Geometry: final body of the model. Coordinates: model frame, mm. A direction names the side the tool comes from. Give positions to 0.01 mm unless a question says otherwise; leave off trailing zeros. Write each loop counter-clockwise with the first axis right and the second up, starting at its lowest first coordinate (ties: lowest second). Pieces come first, ordered by that corner, then holes.
```python
from build123d import *

# Parameters (mm, degrees)
BOSS_EXTRU_1_DEPTH      = 6
ESQUISSE2_W             = 150
ESQUISSE2_H             = 120
BOSS_EXTRU_2_DEPTH      = 6
ESQUISSE3_W             = 6
ESQUISSE3_H             = 50
ESQUISSE3_W_2           = 50
ESQUISSE3_H_2           = 6
ENL_V_MAT_EXTRU_1_DEPTH = 10
ESQUISSE4_W             = 50
ESQUISSE4_H             = 6
ENL_V_MAT_EXTRU_2_DEPTH = 10
ESQUISSE5_W             = 263.306064462
ESQUISSE5_H             = 531.54399855
ENL_V_MAT_EXTRU_5_DEPTH = 10
ESQUISSE9_W             = 6
ESQUISSE9_H             = 75
ESQUISSE9_H_2           = 50
ESQUISSE9_H_3           = 40
ENL_V_MAT_EXTRU_6_DEPTH = 10


with BuildPart() as part:
    # Esquisse1 → Boss.-Extru.1 (new body)
    with BuildSketch(Plane.XY):
        Polygon((-50, 335.901139534), (50, 335.901139534), (255.775862069, 10.507079064), (205, -75.642859016), (-205, -75.642859016), (-255.775862069, 10.507079064), align=None)
        with BuildLine():
            Line((-189.319805153, 31.819805153), (-191.794678888, 34.294678888))
            ThreePointArc((-191.794678888, 34.294678888), (-206, 0), (-191.794678888, -34.294678888))
            Line((-191.794678888, -34.294678888), (-189.319805153, -31.819805153))
            ThreePointArc((-189.319805153, -31.819805153), (-202.5, 0), (-189.319805153, 31.819805153))
        make_face(mode=Mode.SUBTRACT)
        with BuildLine():
            Line((-125.680194847, 31.819805153), (-123.205321112, 34.294678888))
            ThreePointArc((-123.205321112, 34.294678888), (-109, 0), (-123.205321112, -34.294678888))
            Line((-123.205321112, -34.294678888), (-125.680194847, -31.819805153))
            ThreePointArc((-125.680194847, -31.819805153), (-112.5, 0), (-125.680194847, 31.819805153))
        make_face(mode=Mode.SUBTRACT)
        with BuildLine():
            Line((-84.319805153, -31.819805153), (-86.794678888, -34.294678888))
            ThreePointArc((-86.794678888, -34.294678888), (-101, 0), (-86.794678888, 34.294678888))
            Line((-86.794678888, 34.294678888), (-84.319805153, 31.819805153))
            ThreePointArc((-84.319805153, 31.819805153), (-97.5, 0), (-84.319805153, -31.819805153))
        make_face(mode=Mode.SUBTRACT)
        with BuildLine():
            Line((-20.680194847, 31.819805153), (-18.205321112, 34.294678888))
            ThreePointArc((-18.205321112, 34.294678888), (-4, 0), (-18.205321112, -34.294678888))
            Line((-18.205321112, -34.294678888), (-20.680194847, -31.819805153))
            ThreePointArc((-20.680194847, -31.819805153), (-7.5, 0), (-20.680194847, 31.819805153))
        make_face(mode=Mode.SUBTRACT)
        with BuildLine():
            Line((20.680194847, -31.819805153), (18.205321112, -34.294678888))
            ThreePointArc((18.205321112, -34.294678888), (4, 0), (18.205321112, 34.294678888))
            Line((18.205321112, 34.294678888), (20.680194847, 31.819805153))
            ThreePointArc((20.680194847, 31.819805153), (7.5, 0), (20.680194847, -31.819805153))
        make_face(mode=Mode.SUBTRACT)
        with BuildLine():
            Line((84.319805153, 31.819805153), (86.794678888, 34.294678888))
            ThreePointArc((86.794678888, 34.294678888), (101, 0), (86.794678888, -34.294678888))
            Line((86.794678888, -34.294678888), (84.319805153, -31.819805153))
            ThreePointArc((84.319805153, -31.819805153), (97.5, 0), (84.319805153, 31.819805153))
        make_face(mode=Mode.SUBTRACT)
        with BuildLine():
            Line((125.680194847, -31.819805153), (123.205321112, -34.294678888))
            ThreePointArc((123.205321112, -34.294678888), (109, 0), (123.205321112, 34.294678888))
            Line((123.205321112, 34.294678888), (125.680194847, 31.819805153))
            ThreePointArc((125.680194847, 31.819805153), (112.5, 0), (125.680194847, -31.819805153))
        make_face(mode=Mode.SUBTRACT)
        with BuildLine():
            Line((189.319805153, 31.819805153), (191.794678888, 34.294678888))
            ThreePointArc((191.794678888, 34.294678888), (206, 0), (191.794678888, -34.294678888))
            Line((191.794678888, -34.294678888), (189.319805153, -31.819805153))
            ThreePointArc((189.319805153, -31.819805153), (202.5, 0), (189.319805153, 31.819805153))
        make_face(mode=Mode.SUBTRACT)
        with BuildLine():
            Line((-139.294678888, 56.63798851), (-136.819805153, 59.112862244))
            ThreePointArc((-136.819805153, 59.112862244), (-150, 90.932667397), (-136.819805153, 122.752472551))
            Line((-136.819805153, 122.752472551), (-139.294678888, 125.227346285))
            ThreePointArc((-139.294678888, 125.227346285), (-153.5, 90.932667397), (-139.294678888, 56.63798851))
        make_face(mode=Mode.SUBTRACT)
        with BuildLine():
            Line((-70.705321112, 56.63798851), (-73.180194847, 59.112862244))
            ThreePointArc((-73.180194847, 59.112862244), (-60, 90.932667397), (-73.180194847, 122.752472551))
            Line((-73.180194847, 122.752472551), (-70.705321112, 125.227346285))
            ThreePointArc((-70.705321112, 125.227346285), (-56.5, 90.932667397), (-70.705321112, 56.63798851))
        make_face(mode=Mode.SUBTRACT)
        with BuildLine():
            Line((-31.819805153, 122.752472551), (-34.294678888, 125.227346285))
            ThreePointArc((-34.294678888, 125.227346285), (-48.5, 90.932667397), (-34.294678888, 56.63798851))
            Line((-34.294678888, 56.63798851), (-31.819805153, 59.112862244))
            ThreePointArc((-31.819805153, 59.112862244), (-45, 90.932667397), (-31.819805153, 122.752472551))
        make_face(mode=Mode.SUBTRACT)
        with BuildLine():
            Line((34.294678888, 56.63798851), (31.819805153, 59.112862244))
            ThreePointArc((31.819805153, 59.112862244), (45, 90.932667397), (31.819805153, 122.752472551))
            Line((31.819805153, 122.752472551), (34.294678888, 125.227346285))
            ThreePointArc((34.294678888, 125.227346285), (48.5, 90.932667397), (34.294678888, 56.63798851))
        make_face(mode=Mode.SUBTRACT)
        with BuildLine():
            Line((73.180194847, 122.752472551), (70.705321112, 125.227346285))
            ThreePointArc((70.705321112, 125.227346285), (56.5, 90.932667397), (70.705321112, 56.63798851))
            Line((70.705321112, 56.63798851), (73.180194847, 59.112862244))
            ThreePointArc((73.180194847, 59.112862244), (60, 90.932667397), (73.180194847, 122.752472551))
        make_face(mode=Mode.SUBTRACT)
        with BuildLine():
            Line((139.294678888, 56.63798851), (136.819805153, 59.112862244))
            ThreePointArc((136.819805153, 59.112862244), (150, 90.932667397), (136.819805153, 122.752472551))
            Line((136.819805153, 122.752472551), (139.294678888, 125.227346285))
            ThreePointArc((139.294678888, 125.227346285), (153.5, 90.932667397), (139.294678888, 56.63798851))
        make_face(mode=Mode.SUBTRACT)
        with BuildLine():
            Line((-84.319805153, 213.685139948), (-86.794678888, 216.160013682))
            ThreePointArc((-86.794678888, 216.160013682), (-101, 181.865334795), (-86.794678888, 147.570655907))
            Line((-86.794678888, 147.570655907), (-84.319805153, 150.045529641))
            ThreePointArc((-84.319805153, 150.045529641), (-97.5, 181.865334795), (-84.319805153, 213.685139948))
        make_face(mode=Mode.SUBTRACT)
        with BuildLine():
            Line((-20.680194847, 213.685139948), (-18.205321112, 216.160013682))
            ThreePointArc((-18.205321112, 216.160013682), (-4, 181.865334795), (-18.205321112, 147.570655907))
            Line((-18.205321112, 147.570655907), (-20.680194847, 150.045529641))
            ThreePointArc((-20.680194847, 150.045529641), (-7.5, 181.865334795), (-20.680194847, 213.685139948))
        make_face(mode=Mode.SUBTRACT)
        with BuildLine():
            Line((20.680194847, 150.045529641), (18.205321112, 147.570655907))
            ThreePointArc((18.205321112, 147.570655907), (4, 181.865334795), (18.205321112, 216.160013682))
            Line((18.205321112, 216.160013682), (20.680194847, 213.685139948))
            ThreePointArc((20.680194847, 213.685139948), (7.5, 181.865334795), (20.680194847, 150.045529641))
        make_face(mode=Mode.SUBTRACT)
        with BuildLine():
            Line((84.319805153, 150.045529641), (86.794678888, 147.570655907))
            ThreePointArc((86.794678888, 147.570655907), (101, 181.865334795), (86.794678888, 216.160013682))
            Line((86.794678888, 216.160013682), (84.319805153, 213.685139948))
            ThreePointArc((84.319805153, 213.685139948), (97.5, 181.865334795), (84.319805153, 150.045529641))
        make_face(mode=Mode.SUBTRACT)
        with BuildLine():
            Line((-31.819805153, 304.617807345), (-34.294678888, 307.09268108))
            ThreePointArc((-34.294678888, 307.09268108), (-48.5, 272.798002192), (-34.294678888, 238.503323305))
            Line((-34.294678888, 238.503323305), (-31.819805153, 240.978197039))
            ThreePointArc((-31.819805153, 240.978197039), (-45, 272.798002192), (-31.819805153, 304.617807345))
        make_face(mode=Mode.SUBTRACT)
        with BuildLine():
            Line((31.819805153, 304.617807345), (34.294678888, 307.09268108))
            ThreePointArc((34.294678888, 307.09268108), (48.5, 272.798002192), (34.294678888, 238.503323305))
            Line((34.294678888, 238.503323305), (31.819805153, 240.978197039))
            ThreePointArc((31.819805153, 240.978197039), (45, 272.798002192), (31.819805153, 304.617807345))
        make_face(mode=Mode.SUBTRACT)
    extrude(amount=BOSS_EXTRU_1_DEPTH)

    # Esquisse2 → Boss.-Extru.2 (add)
    with BuildSketch(Plane.XY.offset(6)):
        with Locations((0, -135.642859016)):
            Rectangle(ESQUISSE2_W, ESQUISSE2_H)
    extrude(amount=-BOSS_EXTRU_2_DEPTH)

    # Esquisse3 → Enlèv. mat.-Extru.1 (cut)
    with BuildSketch(Plane.XY.offset(6)):
        with Locations((-72, -135.642859016)):
            Rectangle(ESQUISSE3_W, ESQUISSE3_H)
        with Locations((0, -192.642859016)):
            Rectangle(ESQUISSE3_W_2, ESQUISSE3_H_2)
        with Locations((72, -135.642859016)):
            Rectangle(ESQUISSE3_W, ESQUISSE3_H)
    extrude(amount=-ENL_V_MAT_EXTRU_1_DEPTH, mode=Mode.SUBTRACT)

    # Esquisse4 → Enlèv. mat.-Extru.2 (cut)
    with BuildSketch(Plane.XY.offset(6)):
        with Locations((-140, -72.642859016)):
            Rectangle(ESQUISSE4_W, ESQUISSE4_H)
        Polygon((-217.693965517, -54.105374496), (-212.524969232, -51.058822772), (-237.912900267, -7.983853732), (-243.081896552, -11.030405456), align=None)
        Polygon((-229.051724138, 52.766047956), (-223.980647871, 49.559151404), (-170.532372009, 134.077089189), (-175.603448276, 137.283985741), align=None)
        Polygon((-71.653061664, 290.43527409), (-76.724137931, 293.642170642), (-130.172413793, 209.124232857), (-125.101337526, 205.917336306), align=None)
        with Locations((0, 332.901139534)):
            Rectangle(ESQUISSE4_W, ESQUISSE4_H)
        with Locations((140, -72.642859016)):
            Rectangle(ESQUISSE4_W, ESQUISSE4_H)
        Polygon((237.912900267, -7.983853732), (243.081896552, -11.030405456), (217.693965517, -54.105374496), (212.524969232, -51.058822772), align=None)
        Polygon((170.532372009, 134.077089189), (175.603448276, 137.283985741), (229.051724138, 52.766047956), (223.980647871, 49.559151404), align=None)
        Polygon((125.101337526, 205.917336306), (130.172413793, 209.124232857), (76.724137931, 293.642170642), (71.653061664, 290.43527409), align=None)
    extrude(amount=-ENL_V_MAT_EXTRU_2_DEPTH, mode=Mode.SUBTRACT)

    # Esquisse5 → Enlèv. mat.-Extru.5 (cut)
    with BuildSketch(Plane.XY.offset(6)):
        with Locations((131.653032231, 70.129140259)):
            Rectangle(ESQUISSE5_W, ESQUISSE5_H)
    extrude(amount=-ENL_V_MAT_EXTRU_5_DEPTH, mode=Mode.SUBTRACT)

    # Esquisse9 → Enlèv. mat.-Extru.6 (cut)
    with BuildSketch(Plane.XY.offset(6)):
        with Locations((-3, -112.142859016)):
            Rectangle(ESQUISSE9_W, ESQUISSE9_H)
        with Locations((-3, 85.357140984)):
            Rectangle(ESQUISSE9_W, ESQUISSE9_H_2)
        with Locations((-3, 270.357140984)):
            Rectangle(ESQUISSE9_W, ESQUISSE9_H_3)
    extrude(amount=-ENL_V_MAT_EXTRU_6_DEPTH, mode=Mode.SUBTRACT)


solid = part.part
```
Item 1: Pin query (flat end, axial travel): pin 1 Ø10 at (x, y) = (-175.5, -17) entering from -Z; pin 2 Ø1.8 at (x, z) = (-4.5, 3) entering from -Y; pin 3 Ø1.8 at (x, z) = (-71.5, 3.5) entering from +Y; pin 4 Ø3 at (y, z) = (-192.5, 2.5) entering from +X. Return the tip coordinate at first contact, or that it passes through.
Found:
pin 1: stops at z = 0
pin 2: stops at y = -189.64
pin 3: stops at y = 303.33
pin 4: stops at x = -25
Item 2: Section B-B, the plane y = 277. Return the cut outline in (x, z), plus the area to 3 significant figures.
Found:
outline: (-80.15, 0) - (-48.32, 0) - (-48.32, 6) - (-80.15, 6) - close; (-44.8, 0) - (-6, 0) - (-6, 6) - (-44.8, 6) - close
area: 424 mm2
Item 3: Pull-direction query (Y, two-part tool) for faces 1 (the face through (-63.549, 314.476, 2.958)), 2 (the face through (-153.497, 91.466, 2.958)), 3 (the face through (-249.34, -0.41, 2.96)); classes: +Y half, -Y half, draft (parallel to the pull), parting line (faces both ways), or undercut.
Found:
face 1: +Y half
face 2: undercut
face 3: -Y half
Item 4: Line query: L1, parallel to X at y = 155.5, z = 2.25; L2, parallel to X at y = 89, z = 3; L3, parallel to X at y = 156, z = 4. Output: solid intervals per line, ascending.
Found:
L1: x = -164.08 to -93.21, -88.97 to -16.03, -11.79 to 0
L2: x = -199.04 to -153.46, -149.96 to -60.04, -56.54 to -48.46, -44.96 to -6
L3: x = -163.77 to -93.53, -89.32 to -15.68, -11.47 to 0
Item 5: Section A-A, the plane y = 84.5. Return the cut outline in (x, z).
Found:
outline: (-201.88, 0) - (-153.07, 0) - (-153.07, 6) - (-201.88, 6) - close; (-149.54, 0) - (-60.46, 0) - (-60.46, 6) - (-149.54, 6) - close; (-56.93, 0) - (-48.07, 0) - (-48.07, 6) - (-56.93, 6) - close; (-44.54, 0) - (-6, 0) - (-6, 6) - (-44.54, 6) - close
Item 6: Reachability of faces 4 (the face through (-211.26, -65.02, 2.96)), 5 (the face through (-97.497, 181.371, 2.958)) from +Z, -Z, +X, -X, +Y, -Y: full face, straight path, thin tool, end or side. Return the list, or none.
Found:
face 4: +Z, -Z, -X, -Y
face 5: +Z, -Z
Item 7: Section C-C, the plane z = 4.25. State how many separate pieces and enclosed holes the cut face has, plus the area to 3 significant figures.
Found:
separate pieces: 1
enclosed holes: 10
area: 72,600 mm2
Item 8: Section D-D, the plane y = -61. Return the cut outline in (x, z), plus the area to 3 significant figures.
Found:
outline: (-213.63, 0) - (0, 0) - (0, 6) - (-213.63, 6) - close
area: 1,280 mm2
